Could you check a few things on this drawing? It's one solid part, dimensions in mm from its lowest x, y, z. Give positions to 0.01 mm unless a question says otherwise; leave off trailing zeros. Order: outer loops, then holes, each group sorted by start corner. A loop starts at its lowest first (then second) coordinate and runs counter-clockwise, first axis right, second up. Notation, with made-up numbers: (-18.75, 85.5) -> (2.25, 85.5) arc R22 cw to (2.25, 91.5) -> close; hole circle Ø6 at (2.25, -10.5). An arc over 180 degrees is marked (long way). Answer as a JSON object with one key per item and string values.
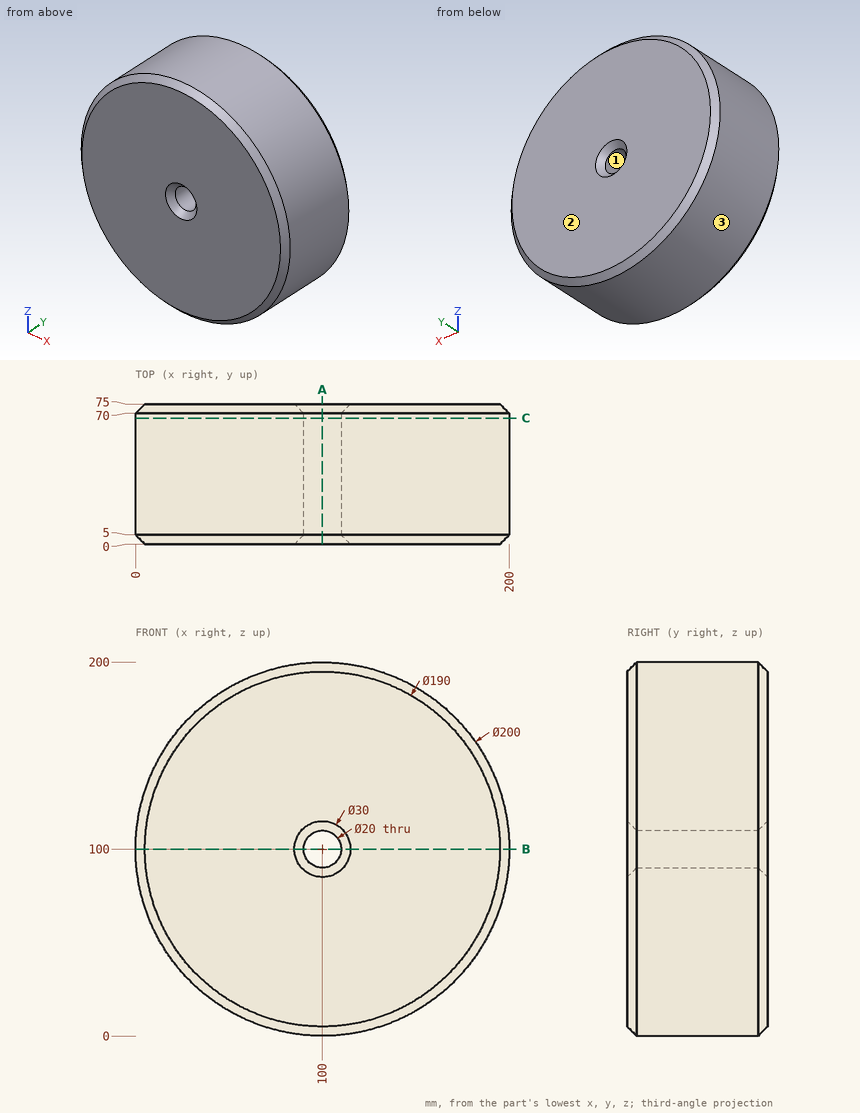
1. Will these pins go through, and if not, where does the flat tip stop? pin 1 Ø1.5 at (x, y) = (62.5, 51.5) entering from -Z; pin 2 Ø2 at (x, y) = (146, 35) entering from +Z; pin 3 Ø3 at (x, y) = (97, 58.5) entering from -Z; pin 4 Ø18 at (x, z) = (100, 100) entering from -Y.
Worked answers:
{"pin 1": "z = 7", "pin 2": "z = 189.3", "pin 3": "z = 0.01", "pin 4": "through"}
2. If we section it at C-C on y = 67.5: Please give me the cut outline in (x, z), then the cut area to 3 significant figures.
Worked answers:
{"outline": "circle Ø200 at (100, 100); hole circle Ø20 at (100, 100)", "area": "31,100 mm²"}
3. If we section it at B-B on z = 100: Please give me the cut outline in (x, y), then the cut area to 3 significant figures.
Worked answers:
{"outline": "(0, 5) -> (5, 0) -> (85, 0) -> (90, 5) -> (90, 70) -> (85, 75) -> (5, 75) -> (0, 70) -> close; (110, 5) -> (115, 0) -> (195, 0) -> (200, 5) -> (200, 70) -> (195, 75) -> (115, 75) -> (110, 70) -> close", "area": "13,400 mm²"}
4. Please list where these lines run through material, in increasing order: L1, parallel to Z at x = 100, y = 27.5; L2, parallel to Z at x = 94.5, y = 31.5; L3, parallel to X at y = 18, z = 102.
Worked answers:
{"L1": "0 to 90, 110 to 200", "L2": "0.15 to 91.65, 108.35 to 199.85", "L3": "0.02 to 90.2, 109.8 to 199.98"}
5. If we mould it in two halves opening along X, with no side actions, what happens to the marked faces 1, 2 and 3? For each: +X half, -X half, draft (parallel to the pull), parting line (faces both ways), or undercut.
Worked answers:
{"face 1": "undercut", "face 2": "draft", "face 3": "parting line"}
6. If we section it at A-A on x = 100: Please give me the cut outline in (y, z), then the cut area to 3 significant figures.
Worked answers:
{"outline": "(0, 5) -> (5, 0) -> (70, 0) -> (75, 5) -> (75, 85) -> (70, 90) -> (5, 90) -> (0, 85) -> close; (0, 115) -> (5, 110) -> (70, 110) -> (75, 115) -> (75, 195) -> (70, 200) -> (5, 200) -> (0, 195) -> close", "area": "13,400 mm²"}
